Geometry: final body of the model. Coordinates: model frame, mm. A direction names the side the tool comes from. Round coordinates to 2 decimals unless told otherwise and drop trailing zeros. Write each loop counter-clockwise with the first axis right and the second up, starting at its lowest first coordinate (ties: lowest second). Pieces come first, ordered by that corner, then holes. Notation, with made-up numbers: M 6,67.5 L 57,67.5 A18 ccw 57,99.5 Z; hole C 21.5,33.5 d3. An arc over 180 degrees is marked long. Use one line per item in the form item = value. Start each with the question number.
Item 1: Pin query (flat end, axial travel): pin 1 Ø6.5 at (x, y) = (-17.5, -44) entering from +Z; pin 2 Ø7.5 at (x, y) = (-181, -20) entering from +Z; pin 3 Ø7.5 at (x, z) = (114.3, 12.7) entering from -Y. Return the tip coordinate at first contact, or that it passes through.
Item 2: Section query A-A (z = -4.5). Return loops of the section in (x, y).
Item 3: Ray query, probe 1 along X at (y, z) = (-3, 12); probe 2 along Y at (x, z) = (177, -10.5); probe 3 along Z at (x, y) = (342.9, -7) (3 decimals). Return the intervals inside material, ascending.
Item 4: Pull-direction query (Y, two-part tool) for faces 3 (the flat face through (-6, -50.8, -10)), 4 (the flat face through (-6, -25, -12.7)), 5 (the flat face through (-6, -38.1, -3)), 6 (the flat face through (-457.2, -20, -17)); classes: pulls with the +Y half, pulls with the -Y half, needs draft (parallel to the pull), parting line crosses it, or undercut.
Item 5: Section query B-B (x = 137). Return loops of the section in (y, z), and give its area (3 significant figures).
Item 6: Reachability of faces 1 (the flat face through (-6, -12.7, 7)), 2 (the flat face through (-6, -25, -25.4)) from +Z, -Z, +X, -X, +Y, -Y: full face, straight path, thin tool, end or side. Return the list, or none.
from build123d import *

# Parameters (mm, degrees)
F0_W     = 914.4
F0_H     = 50.8
F1_DEPTH = 12.7
F2_W     = 914.4
F2_H     = 12.7
F3_DEPTH = 38.1
F4_W     = 914.4
F4_H     = 12.7
F5_DEPTH = 19.05
F7_D     = 6.35


with BuildPart() as f1:
    # F0 (on Front) → F1 (new body)
    with BuildSketch(Plane.XZ):
        Rectangle(F0_W, F0_H)
    extrude(amount=F1_DEPTH)

    # F2 (on face) → F3 (join)
    with BuildSketch(Plane.XZ.offset(12.7)):
        with Locations((0, -19.05)):
            Rectangle(F2_W, F2_H)
    extrude(amount=F3_DEPTH)

    # F4 (on face) → F5 (join)
    with BuildSketch(Plane.XY.offset(-12.7)):
        with Locations((0, -44.45)):
            Rectangle(F4_W, F4_H)
    extrude(amount=F5_DEPTH)

    # F7 (through all)
    with Locations(Plane.XZ.offset(12.7)):
        with Locations((-342.9, 12.7), (-114.3, 12.7), (114.3, 12.7), (342.9, 12.7)):
            Hole(F7_D / 2)


solid = f1.part
Working result:
q1.pin_1 = 6.35
q1.pin_2 = -12.7
q1.pin_3 = -12.7
q2.outline = M -457.2,-50.8 L 457.2,-50.8 L 457.2,-38.1 L -457.2,-38.1 Z; M -457.2,-12.7 L 457.2,-12.7 L 457.2,0 L -457.2,0 Z
q3.probe_1 = -457.2 to -346, -339.8 to -117.4, -111.2 to 111.2, 117.4 to 339.8, 346 to 457.2
q3.probe_2 = -50.8 to -38.1, -12.7 to 0
q3.probe_3 = -25.4 to 9.525, 15.875 to 25.4
q4.face_3 = pulls with the -Y half
q4.face_4 = undercut
q4.face_5 = undercut
q4.face_6 = needs draft
q5.outline = M -50.8,-25.4 L 0,-25.4 L 0,25.4 L -12.7,25.4 L -12.7,-12.7 L -38.1,-12.7 L -38.1,6.35 L -50.8,6.35 Z
q5.area = 1,370 mm²
q6.face_1 = +Z, +X, -X
q6.face_2 = -Z, +X, -X, +Y, -Y
